Verification items for the finished model (mm, model axes). A direction names the side the tool comes from. Give positions to 0.01 mm unless a question says otherwise; leave off trailing zeros. Order: outer loops, then holes, each group sorted by start corner. A loop starts at its lowest first (then second) coordinate and runs counter-clockwise, first axis right, second up. Notation, with made-up numbers: M 2.5,-22 L 12.5,-22 A28 ccw 12.5,2 Z; hole C -34,78 d3. An arc over 180 degrees is marked long. Answer as a JSON object with one key per item and string values.
```python
from build123d import *

# Parameters (mm, degrees)
F0_W     = 81.449031
F0_H     = 71.375828
F1_DEPTH = 50.8
F2_W     = 20.32
F2_H     = 8.815292
F2_R     = 2.947041
F2_H_2   = 9.711764
F2_R_2   = 2.935696
F2_W_2   = 10.757647
F2_H_3   = 5.827058
F3_DEPTH = 0.254
F4_SIZE  = 5.08
F5_SIZE  = 5.08
F6_R     = 2.413
F7_DEPTH = 12.7


with BuildPart() as f1:
    # F0 (on Top) → F1 (new body)
    with BuildSketch(Plane.XY):
        with Locations((2.302446, 3.885379)):
            Rectangle(F0_W, F0_H)
    extrude(amount=F1_DEPTH)

    # F2 (on face) → F3 (join)
    with BuildSketch(Plane.XZ.offset(31.802535)):
        with Locations((-15.56207, 39.818236)):
            Rectangle(F2_W, F2_H)
        with Locations((-18.825882, 40.044982)):
            Circle(F2_R, mode=Mode.SUBTRACT)
        with Locations((20.166961, 39.668823)):
            Rectangle(F2_W, F2_H_2)
        with Locations((17.481177, 39.596712)):
            Circle(F2_R_2, mode=Mode.SUBTRACT)
        with Locations((0.298823, 27.566471)):
            Rectangle(F2_W_2, F2_H_3)
        Polygon((-22.112939, 16.584706), (-26.296471, 20.32), (-26.296471, 3.287059), (-22.877605, 7.272481), (-18.23174, 3.287059), (-15.538824, 8.516526), (-11.504705, 3.287059), (-9.26353, 8.66595), (-6.125882, 3.287059), (-4.631764, 8.217677), (0, 4.244351), (1.643529, 8.367102), (6.125882, 3.287059), (10.336007, 8.194863), (12.849411, 3.287059), (17.048708, 8.182241), (21.067059, 3.287059), (22.710588, 8.66595), (26.744705, 3.287059), (28.687059, 9.263645), (32.870589, 3.287059), (34.812941, 10.309614), (34.812941, 15.389412), (30.928233, 20.32), (29.135293, 16.584706), (25.250589, 20.32), (24.052847, 16.584706), (19.495787, 20.32), (16.43407, 16.584706), (11.877011, 20.32), (8.815294, 16.584706), (4.258235, 20.32), (2.926819, 16.584706), (-1.427469, 20.32), (-4.631764, 16.584706), (-8.986052, 20.32), (-14.215461, 16.584706), (-16.88353, 20.32), align=None)
        Polygon((-16.88353, 20.32), (-26.296471, 20.32), (-22.112939, 16.584706), align=None)
        Polygon((-8.986052, 20.32), (-16.88353, 20.32), (-14.215461, 16.584706), align=None)
        Polygon((-22.877605, 7.272481), (-26.296471, 3.287059), (-18.23174, 3.287059), align=None)
        Polygon((-1.427469, 20.32), (-8.986052, 20.32), (-4.631764, 16.584706), align=None)
        Polygon((-15.538824, 8.516526), (-18.23174, 3.287059), (-11.504705, 3.287059), align=None)
        Polygon((4.258235, 20.32), (-1.427469, 20.32), (2.926819, 16.584706), align=None)
        Polygon((-9.26353, 8.66595), (-11.504705, 3.287059), (-6.125882, 3.287059), align=None)
        Polygon((11.877011, 20.32), (4.258235, 20.32), (8.815294, 16.584706), align=None)
        Polygon((-4.631764, 8.217677), (-6.125882, 3.287059), (6.125882, 3.287059), (1.643529, 8.367102), (0, 4.244351), align=None)
        Polygon((19.495787, 20.32), (11.877011, 20.32), (16.43407, 16.584706), align=None)
        Polygon((10.336007, 8.194863), (6.125882, 3.287059), (12.849411, 3.287059), align=None)
        Polygon((25.250589, 20.32), (19.495787, 20.32), (24.052847, 16.584706), align=None)
        Polygon((17.048708, 8.182241), (12.849411, 3.287059), (21.067059, 3.287059), align=None)
        Polygon((30.928233, 20.32), (25.250589, 20.32), (29.135293, 16.584706), align=None)
        Polygon((22.710588, 8.66595), (21.067059, 3.287059), (26.744705, 3.287059), align=None)
        Polygon((34.812941, 20.32), (30.928233, 20.32), (34.812941, 15.389412), align=None)
        Polygon((28.687059, 9.263645), (26.744705, 3.287059), (32.870589, 3.287059), align=None)
        Polygon((34.812941, 10.309614), (32.870589, 3.287059), (34.812941, 3.287059), align=None)
    extrude(amount=F3_DEPTH)

    # F4
    f4_edges = [f1.edges().sort_by_distance(p)[0] for p in [
        (2.302445, -31.802535, 50.8),
        (-38.42207, -31.802535, 25.4),
        (43.026961, -31.802535, 25.4),
    ]]
    chamfer(f4_edges, length=F4_SIZE)

    # F5
    f5_edges = [f1.edges().sort_by_distance(p)[0] for p in [
        (-38.42207, 6.425379, 50.8),
        (43.026961, 6.425379, 50.8),
        (2.302445, 39.573293, 50.8),
    ]]
    chamfer(f5_edges, length=F5_SIZE)

    # F6 (on face) → F7 (cut)
    with BuildSketch(Plane(origin=(0, 0, 0), x_dir=(1, 0, 0), z_dir=(0, 0, -1))):
        Circle(F6_R)
    extrude(amount=-F7_DEPTH, mode=Mode.SUBTRACT)


solid = f1.part
```
Q1. Section check A-A on y = 0. Record the cut outline in (x, z), then the cut area to 3 significant figures.
Resolved:
{"outline": "M -38.42,0 L -2.41,0 L -2.41,12.7 L 2.41,12.7 L 2.41,0 L 43.03,0 L 43.03,45.72 L 37.95,50.8 L -33.34,50.8 L -38.42,45.72 Z", "area": "4,050 mm²"}
Q2. Release check for a two-part mould opening along X. For faces 1 (the face through (4, -32.057, 12)), 2 (the face through (-1.915, 1.468, 6.261)), 3 (the face through (-35.847, 4.674, 48.296)) record: +X half, -X half, draft (parallel to the pull), parting line (faces both ways), or undercut.
Resolved:
{"face 1": "draft", "face 2": "undercut", "face 3": "-X half"}
Q3. Section check B-B on x = 0. Record the cut outline in (y, z).
Resolved:
{"outline": "M -32.06,3.29 L -31.8,3.29 L -31.8,0 L -2.41,0 L -2.41,12.7 L 2.41,12.7 L 2.41,0 L 39.57,0 L 39.57,45.72 L 34.49,50.8 L -26.72,50.8 L -31.8,45.72 L -31.8,30.48 L -32.06,30.48 L -32.06,24.65 L -31.8,24.65 L -31.8,20.32 L -32.06,20.32 Z"}
Q4. Gauge pin test, flat end, axial feed: pin 1 Ø3.5 at (x, z) = (17.48, 39.6) entering from -Y. Record the tip position at first contact, or that the pin passes through.
Resolved:
{"pin 1": "stops at y = -31.8"}
Q5. Section check C-C on z = 47. Record the cut outline in (x, y).
Resolved:
{"outline": "M -37.14,-28 L -34.62,-30.52 L 39.23,-30.52 L 41.75,-28 L 41.75,38.29 L -37.14,38.29 Z"}
Q6. Tool access check on faces 4 (the face through (17, -31.803, 40)), 5 (the face through (0, 0, 12.7)), 6 (the face through (43.027, 6, 23)). Record the directions out of +Z, -Z, +X, -X, +Y, -Y that give a thin tool (end or side, any length) a straight path to the whole face; none if there is none.
Resolved:
{"face 4": "-Y", "face 5": "-Z", "face 6": "+Z, -Z, +X, +Y, -Y"}
Q7. Material ranges on L1, parallel to Y at x = 0, z = 7; L2, parallel to Y at x = 33, z = 42.5; L3, parallel to X at y = 0, z = 7.75, recorded low to high.
Resolved:
{"L1": "y = -32.06 to -2.41, 2.41 to 39.57", "L2": "y = -31.8 to 39.57", "L3": "x = -38.42 to -2.41, 2.41 to 43.03"}
